Autodesk Inventor part; units mm, degrees
ref_plane "Arbeitsebene1" through (-69, 0, -78.309) normal (0, -0.0498957, -0.9987544) x (1, 0, 0)
ref_plane "YZ Plane" through (0, 0, 0) normal (1, 0, 0) x (0, 1, 0)
ref_plane "XZ Plane" through (0, 0, 0) normal (0, 1, 0) x (-1, 0, 0)
sketch "Skizze1" plane through (0, 0, 0) normal (0, 1, 0) x (-1, 0, 0)
  line L0 (0, 0) -> (69, 0)
  line L1 (69, 0) -> (69, -78.309)
  line L2 (69, -78.309) -> (0, -78.309)
  line L3 (0, -78.309) -> (0, 0)
  dimension "d0" = 69
  dimension "d1" = 78.309
extrude "Extrusion1" add sketch "Skizze1" against normal blind 3
ref_plane "Arbeitsebene1" through (-69, 0, -78.309) normal (0, -0.0498957, -0.9987544) x (1, 0, 0)
sketch "Skizze2" plane through (-69, 0, -78.309) normal (0, -0.0498957, -0.9987544) x (1, 0, 0)
  line L0 (0, 0) -> (69, 0)
  line L1 (69, 0) -> (69, 2.9963)
  line L2 (0, 2.9963) -> (69, 2.9963)
  line L3 (0, 0) -> (0, 2.9963)
  line L4 (69, 0) -> (0, 0)
  line L5 (0, 0) -> (0, -67.1)
  line L6 (0, -67.1) -> (69, -67.1)
  line L7 (69, -67.1) -> (69, 0)
  point P0 (69, 3.9073)
  dimension "d5" = 69
  dimension "d6" = 67.1
extrude "Extrusion2" add sketch "Skizze2" along normal blind 4 contours L0 L7 L6 L5
sketch "Skizze4" plane through (-69, 0, -78.309) normal (0, 0.0498957, 0.9987544) x (1, 0, 0)
  line L0 (0, 0) -> (0, 67.1)
  line L1 (0, 67.1) -> (69, 67.1)
  line L2 (69, 67.1) -> (69, 0)
  line L3 (0, 0) -> (69, 0)
  line L4 (69, 67.1) -> (69, 0)
  line L5 (0, 67.1) -> (69, 67.1)
  line L6 (0, 0) -> (0, 67.1)
  line L7 (69, 0) -> (0, 0)
  point P0 (69, -3.9073)
  point P1 (61.5, 59.466)
  point P2 (7.5, 59.466)
  dimension "d12" = 7.634
  dimension "d14" = 7.5
  dimension "d15" = 7.634
  dimension "d16" = 7.5
hole "Bohrung1" at (-7.5, 59.3919, -81.2761) at (-61.5, 59.3919, -81.2761) direction (0, -0.0498957, -0.9987544) diameter 3 depth 8 tip angle 118
sketch "Skizze5" plane through (0, 0, 0) normal (0, 1, 0) x (1, 0, 0)
  line L0 (0, 0) -> (-69, 0)
  line L1 (0, 78.309) -> (0, 0)
  line L2 (-69, 78.309) -> (0, 78.309)
  line L3 (-69, 0) -> (-69, 78.309)
  line L4 (-10, 62.9) -> (-45.1, 62.9)
  line L5 (-45.1, 62.9) -> (-45.1, 15.9)
  line L6 (-45.1, 15.9) -> (-10, 15.9)
  line L7 (-10, 15.9) -> (-10, 62.9)
  line L8 (-5, 66.4) -> (-51, 66.4)
  line L9 (-51, 66.4) -> (-51, 12.4)
  line L10 (-51, 12.4) -> (-5, 12.4)
  line L11 (-5, 12.4) -> (-5, 66.4)
  circle A0 centre (-59, 12) radius 5
  circle A1 centre (-56, 49.009) radius 3.5
  point P0 (-5, 2.588)
  point P1 (-65, 2.588)
  dimension "d24" = 35.1
  dimension "d25" = 47
  dimension "d26" = 54
  dimension "d27" = 46
  dimension "d28" = 5
  dimension "d29" = 3.5
  dimension "d30" = 12.4
  dimension "d31" = 5
  dimension "d32" = 7
  dimension "d34" = 13
  dimension "d35" = 10
  dimension "d37" = 10
  dimension "d40" = 5
  dimension "d41" = 2.588
  dimension "d42" = 4
  dimension "d56" = 29.3
  dimension "d57" = 12
extrude "Extrusion4" cut sketch "Skizze5" against normal blind 69 contours L7 L6 L5 L4 | A0 | A1
extrude "Extrusion5" cut sketch "Skizze5" against normal blind 1.5 contours L11 L10 L9 L8
hole "Bohrung2" at (-5, 0, -2.588) at (-65, 0, -2.588) direction (0, -1, 0) diameter 3 depth 8 tip angle 118
sketch "Skizze6" plane through (0, 0, -78.309) normal (1, 0, 0) x (0, -0.0498957, -0.9987544)
  line L0 (0, 0) -> (0.1497, -2.9963)
  line L1 (0, 0) -> (-78.2115, -3.9073)
  line L2 (-78.2115, -3.9073) -> (-78.0618, -6.9035)
  line L3 (0.1497, -2.9963) -> (-78.0618, -6.9035)
  line L4 (0, 0) -> (0.1497, -2.9963)
  line L5 (0, 67.1) -> (0, 0)
  line L6 (0, 0) -> (4, 0)
  line L7 (4, 67.1) -> (4, 0)
  line L8 (0, 67.1) -> (4, 67.1)
  line L9 (4, 0) -> (0, 0)
  line L10 (0, 0) -> (4, 0)
  line L11 (0, 0) -> (0.1497, -2.9963)
  line L12 (0.1497, -2.9963) -> (4, -2.8039)
  line L13 (4, -2.8039) -> (4, 0)
  line L14 (0.1497, -2.9963) -> (-78.0618, -6.9035)
  point P0 (4, 0)
extrude "Extrusion6" add sketch "Skizze6" against normal blind 69 contours L6 L13 L12 L0
sketch "Skizze7" plane through (-69, -3, 0) normal (-1, 0, 0) x (0, 0, 1)
  line L0 (0, 3) -> (-78.309, 3)
  line L1 (-78.309, 3) -> (-81.657, 70.0164)
  line L2 (-81.657, 70.0164) -> (-85.652, 69.8168)
  line L3 (-85.652, 69.8168) -> (-82.1641, 0)
  line L4 (0, 0) -> (-82.1641, 0)
  line L5 (0, 3) -> (0, 0)
  line L6 (-78.309, 3) -> (-81.657, 70.0164)
  line L7 (-85.652, 69.8168) -> (-82.1641, 0)
  line L8 (-85.5985, 68.7464) -> (-81.657, 70.0164)
  line L9 (0, 0) -> (0, 3)
  line L10 (0, 0) -> (0, 3)
  line L11 (0, 3) -> (0.8038, 0)
  line L12 (0.8038, 0) -> (0, 0)
  line L13 (0.8038, 0) -> (0, 0)
  line L14 (0, 0) -> (0, 3)
  line L15 (0, 3) -> (0.8038, 3)
  line L16 (0.8038, 3) -> (0.8038, 0)
  line L17 (0, 0) -> (0, 3)
  line L18 (0, 3) -> (0, 0)
  point P0 (-0.4568, 4.2362)
  dimension "d59" = 15
  dimension "d62" = 15
extrude "Extrusion7" cut sketch "Skizze7" against normal blind 80 contours L8 L3 L2
extrude "Extrusion8" add sketch "Skizze7" against normal blind 69 contours L11 L12 L5
properties part number "Dekel"
Design review of the part built by this model. Coordinates are the model's own, in mm. A direction names the side the tool comes from. Give positions to 0.01 mm unless a question says otherwise; leave off trailing zeros. Write each loop counter-clockwise with the first axis right and the second up, starting at its lowest first coordinate (ties: lowest second). Pieces come first, ordered by that corner, then holes. Notation, with made-up numbers: (49, 24) -> (88, 24) arc R22 ccw to (88, 51) -> close; hole circle Ø9 at (49, -16.5). An arc over 180 degrees is marked (long way). Answer in a Markdown table with one row per item.
(1) To check wall thickness, follow probe 1 along Z at (x, y) = (-59, -1); probe 2 along Z at (x, y) = (-56, -1); probe 3 along X at (y, z) = (-2, -12). State the ranges of each line that lie inside material, in increasing order.
Results:
| item | result |
|---|---|
| probe 1 | -82.26 to -50.81, -47.21 to -17, -7 to 0.27 |
| probe 2 | -82.26 to -52.51, -45.51 to -16, -8 to 0.27 |
| probe 3 | -69 to -64, -54 to 0 |
(2) Consider section D-D (y = 10.5). State the section outline as (x, z) points.
Results:
| item | result |
|---|---|
| outline | (-69, -82.84) -> (0, -82.84) -> (0, -78.83) -> (-69, -78.83) -> close |
(3) For faces 4 (the flat face through (-57, 0, -39)), 5 (the cylindrical face through (-66.265, -1.521, -1.782)), 6 (the flat face through (-8, -1.5, -40)), list the 3-axis set-ups (+Z, -Z, +X, -X, +Y, -Y) from which the entire face can be reached by the end or side of a thin tool; tool diameter is ignored.
Results:
| item | result |
|---|---|
| face 4 | +Z, +X, -X, +Y |
| face 5 | +Y, -Y |
| face 6 | +Y |
(4) Consider section A-A (x = -56). State the section outline as (y, z) points, then the cut area to 3 significant figures.
Results:
| item | result |
|---|---|
| outline | (-3, -82.16) -> (65.75, -85.6) -> (67.02, -81.66) -> (0, -78.31) -> (0, -52.51) -> (-3, -52.51) -> (-3, -78.31) -> close; (-3, -45.51) -> (0, -45.51) -> (0, -16) -> (-3, -16) -> close; (-3, -8) -> (0, -8) -> (0, 0) -> (-3, 0.8) -> close |
| area | 469 mm2 |
(5) Mouldability with a two-part tool opening along X and no side actions: class faces 1 (the flat face through (0, 19, -81)), 2 (the flat face through (-34.98, 66.37, -83.66)), 3 (the cylindrical face through (-62.765, 58.485, -83.261)) as +X half, -X half, draft (parallel to the pull), parting line (faces both ways), or undercut.
Results:
| item | result |
|---|---|
| face 1 | +X half |
| face 2 | draft |
| face 3 | undercut |
(6) Consider section C-C (x = -32). State the section outline as (y, z) points, then the cut area to 3 significant figures.
Results:
| item | result |
|---|---|
| outline | (-3, -82.16) -> (65.75, -85.6) -> (67.02, -81.66) -> (0, -78.31) -> (0, -66.4) -> (-1.5, -66.4) -> (-1.5, -62.9) -> (-3, -62.9) -> (-3, -78.31) -> close; (-3, -15.9) -> (-1.5, -15.9) -> (-1.5, -12.4) -> (0, -12.4) -> (0, 0) -> (-3, 0.8) -> close |
| area | 362 mm2 |
(7) Clearance check with flat-ended pins moving along their axes: pin 1 (0.8 mm diameter, centred on x = -22, y = -0.5, fed in from +Z); pin 2 (4 mm diameter, centred on x = -65, z = -2.588, fed in from -Y); pin 3 (1 mm diameter, centred on x = -60, z = -48.5, fed in from +Y); pin 4 (0.8 mm diameter, centred on x = -31, y = -2.5, fed in from -Z). State where each tip first meets the part, or that it passes through.
Results:
| item | result |
|---|---|
| pin 1 | z = 0.24 |
| pin 2 | y = -3 |
| pin 3 | y = 0 |
| pin 4 | z = -82.21 |
(8) Consider section B-B (z = -21.5). State the section outline as (x, y) points, then the cut area to 4 significant figures.
Results:
| item | result |
|---|---|
| outline | (-69, -3) -> (-45.1, -3) -> (-45.1, -1.5) -> (-51, -1.5) -> (-51, 0) -> (-69, 0) -> close; (-10, -3) -> (0, -3) -> (0, 0) -> (-5, 0) -> (-5, -1.5) -> (-10, -1.5) -> close |
| area | 85.35 mm2 |
